Autodesk Inventor part; units mm, degrees
ref_plane "YZ Plane" through (0, 0, 0) normal (1, 0, 0) x (0, 1, 0)
ref_plane "XZ Plane" through (0, 0, 0) normal (0, 1, 0) x (-1, 0, 0)
ref_plane "XY Plane" through (0, 0, 0) normal (0, 0, 1) x (1, 0, 0)
sketch "Esquisse12" plane through (0, 0, 0) normal (0, 0, 1) x (1, 0, 0)
  line L0 (0, 0) -> (20, 0)
  line L1 (20, 0) -> (20, 38)
  line L2 (20, 38) -> (0, 38)
  line L3 (0, 38) -> (0, 0)
  line L4 (10, 38) -> (10, 0) construction
  circle A0 centre (10, 7) radius 2.15
  line L5 (10, 7) -> (20, 7) construction
  circle A1 centre (16, 7) radius 2.15
  circle A2 centre (4, 7) radius 2.15
  circle A3 centre (10, 7) radius 2.15
  circle A4 centre (10, 25) radius 2.15
  circle A5 centre (16, 25) radius 2.15
  circle A6 centre (4, 25) radius 2.15
  dimension "d133" = 20
  dimension "d134" = 7
  dimension "d135" = 4.3
  dimension "d138" = 6
  dimension "d141" = 6
  dimension "d148" = 18
  dimension "d153" = 13
extrude "Extrusion13" add sketch "Esquisse12" along normal blind 2.2
fillet "Congé8" radius 7 2 edges at (20, 0, 1.1) (0, 0, 1.1)
mirror "Symétrie3" about plane through (20, 38, 0) normal (0, 1, 0)
equation "\"d135\" = Holes"
equation "\"d154\" = Depth"
equation "\"d156\" = Rounding"
equation "\"Depth\" = 2.2"
equation "\"Holes\" = 4.3"
equation "\"Height\" = 0"
equation "\"Rounding\" = 7"
properties part number "SideToSide"
Verification items for the finished model (mm, model axes). Coordinates: 2 decimals unless noted, no trailing zeros. Order: outer loops, then holes, each group sorted by start corner. A loop starts at its lowest first (then second) coordinate and runs counter-clockwise, first axis right, second up. Notation, with made-up numbers: (67, -36) -> (82, -36) arc R25 ccw to (82, -9) -> close; hole circle Ø9 at (57, 4). An arc over 180 degrees is marked (long way). Put each result on its own line as item: value. Start each with the question number.
1) Cross-section at D-D (x = 16.5). Enter the section's corners in (y, z), plus the area to 3 significant figures.
2) Cross-section at C-C (z = 1.85). State how many separate pieces and enclosed holes the cut face has, plus the area to 3 significant figures.
3) Cross-section at A-A (x = 10). Enter the section's corners in (y, z).
4) Material ranges on L1, parallel to X at y = 69, z = 1.35; L2, parallel to Y at x = 10, z = 1.65; L3, parallel to Y at x = 16, z = 1.7, recorded low to high.
5) Release check for a two-part mould opening along Y. For faces 1 (the cylindrical face through (18, 73.9, 1.1)), 2 (the cylindrical face through (3.72, 48.87, 1.08)), 3 (the flat face through (10, 39, 2.2)), 4 (the cylindrical face through (9.72, 4.87, 1.08)) record: pulls with the +Y half, pulls with the -Y half, needs draft (parallel to the pull), parting line crosses it, or undercut.
6) Cross-section at B-B (y = 25). Enter the section's corners in (x, z).
Geometry check:
1. outline: (0.94, 0) -> (4.91, 0) -> (4.91, 2.2) -> (0.94, 2.2) -> close; (9.09, 0) -> (22.91, 0) -> (22.91, 2.2) -> (9.09, 2.2) -> close; (27.09, 0) -> (48.91, 0) -> (48.91, 2.2) -> (27.09, 2.2) -> close; (53.09, 0) -> (66.91, 0) -> (66.91, 2.2) -> (53.09, 2.2) -> close; (71.09, 0) -> (75.06, 0) -> (75.06, 2.2) -> (71.09, 2.2) -> close
1. area: 126 mm^2
2. separate pieces: 1
2. enclosed holes: 12
2. area: 1,300 mm^2
3. outline: (0, 0) -> (4.85, 0) -> (4.85, 2.2) -> (0, 2.2) -> close; (9.15, 0) -> (22.85, 0) -> (22.85, 2.2) -> (9.15, 2.2) -> close; (27.15, 0) -> (48.85, 0) -> (48.85, 2.2) -> (27.15, 2.2) -> close; (53.15, 0) -> (66.85, 0) -> (66.85, 2.2) -> (53.15, 2.2) -> close; (71.15, 0) -> (76, 0) -> (76, 2.2) -> (71.15, 2.2) -> close
4. L1: x = 0 to 1.85, 6.15 to 7.85, 12.15 to 13.85, 18.15 to 20
4. L2: y = 0 to 4.85, 9.15 to 22.85, 27.15 to 48.85, 53.15 to 66.85, 71.15 to 76
4. L3: y = 0.68 to 4.85, 9.15 to 22.85, 27.15 to 48.85, 53.15 to 66.85, 71.15 to 75.32
5. face 1: pulls with the +Y half
5. face 2: undercut
5. face 3: needs draft
5. face 4: undercut
6. outline: (0, 0) -> (1.85, 0) -> (1.85, 2.2) -> (0, 2.2) -> close; (6.15, 0) -> (7.85, 0) -> (7.85, 2.2) -> (6.15, 2.2) -> close; (12.15, 0) -> (13.85, 0) -> (13.85, 2.2) -> (12.15, 2.2) -> close; (18.15, 0) -> (20, 0) -> (20, 2.2) -> (18.15, 2.2) -> close
